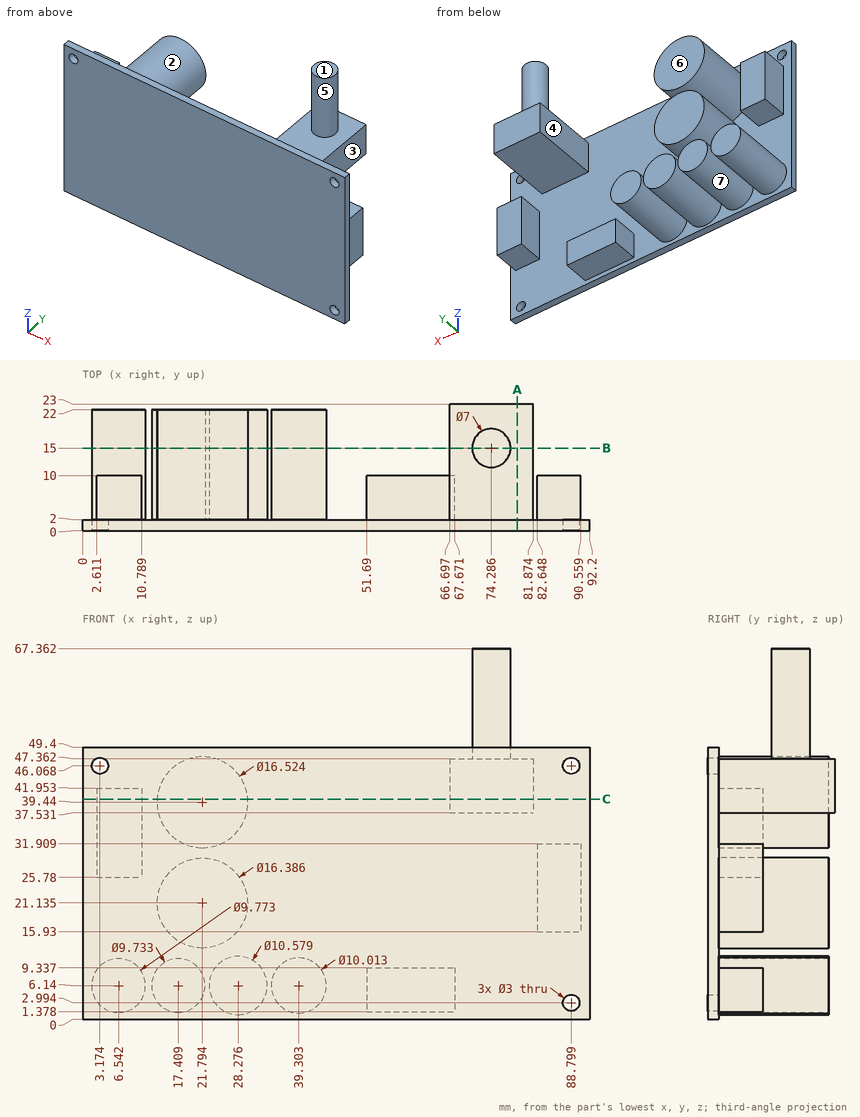
Geometry check sheet. Reference: drawing and pictorial views, mm from the part's lowest x, y, z. A direction names the side the tool comes from. Give positions to 0.01 mm unless a question says otherwise; leave off trailing zeros. Write each loop counter-clockwise with the first axis right and the second up, starting at its lowest first coordinate (ties: lowest second). Pieces come first, ordered by that corner, then holes.
Item 1: Cross-section at B-B (y = 15). Count the separate pieces of the cut face and the enclosed holes in it, and give its area (3 significant figures).
Item 2: Draft check along X on the marked faces 1, 2 and 3. Enter one of: released by +X, released by -X, zero draft, split by the parting line, or undercut.
Item 3: Gauge pin test, flat ends, axial feed: pin 1 (8 mm diameter, centred on y = 19, z = 58.5, fed in from +X); pin 2 (8.5 mm diameter, centred on x = 27.5, z = 7, fed in from +Y); pin 3 (1.5 mm diameter, centred on y = 4, z = 13.5, fed in from -X) (1 decimal); pin 4 (2.5 mm diameter, centred on x = 88.8, z = 2.99, fed in from -Y). Record the tip position at first contact, or that the pin passes through.
Item 4: Access from +Z, -Z, +X, -X, +Y, -Y to the whole of each face (thin tool, end or side, straight path). Record for the marked faces 4, 5, 6 and 7.
Item 5: Cross-section at A-A (x = 79). Enter the section's corners in (y, z).
Item 6: Scan lines: L1, parallel to Z at x = 19, y = 21.75 (1 decimal); L2, parallel to Z at x = 14.5, y = 13 (1 decimal); L3, parallel to Y at x = 78, z = 21. Record each from-to range of solid material in increasing order.
Item 7: Cross-section at C-C (z = 40). Enter the section's corners in (x, y) (1 decimal).
Report:
1. separate pieces: 7
1. enclosed holes: 0
1. area: 1,030 mm2
2. face 1: zero draft
2. face 2: undercut
2. face 3: released by +X
3. pin 1: stops at x = 77.79
3. pin 2: stops at y = 22
3. pin 3: stops at x = 17.4
3. pin 4: passes through
4. face 4: +Z, +Y
4. face 5: +Z
4. face 6: +Z, -Z, -X, +Y
4. face 7: +Y
5. outline: (0, 0) - (2, 0) - (2, 37.53) - (23, 37.53) - (23, 47.36) - (2, 47.36) - (2, 49.4) - (0, 49.4) - close
6. L1: z = 1.5 to 10.7, 13.4 to 28.8, 31.7 to 47.2
6. L2: z = 2.2 to 10, 17.4 to 24.9, 35.6 to 43.3
6. L3: y = 0 to 2
7. outline: (0, 0) - (92.2, 0) - (92.2, 2) - (81.9, 2) - (81.9, 23) - (66.7, 23) - (66.7, 2) - (30, 2) - (30, 22) - (13.6, 22) - (13.6, 2) - (10.8, 2) - (10.8, 10) - (2.6, 10) - (2.6, 2) - (0, 2) - close
